Part model, mm, in its own coordinate system. Face numbers are marked on the shaded views. A direction names the side the tool comes from. Give positions to 0.01 mm unless a question says otherwise; leave off trailing zeros. Order: outer loops, then holes, each group sorted by start corner. A loop starts at its lowest first (then second) coordinate and runs counter-clockwise, first axis right, second up.
1. Drop flat-ended pins along their axis: pin 1 Ø2.5 at (x, z) = (-26.5, 0) entering from -Y; pin 2 Ø8 at (x, z) = (1, 2.5) entering from -Y; pin 3 Ø1.5 at (y, z) = (4, -1.5) entering from -X; pin 4 Ø4 at (x, z) = (-13.25, -22.95) entering from +Y. Give the stop position or say it passes through.
2. Slice it at A-A on y = 2. Give the number of separate pieces and of enclosed holes in the cut face, and give its area (3 significant figures).
3. Slice it at B-B on x = -26.5. List the corners of the cut face in (y, z).
4. Mould opens along X. For the marked faces 1 and 2 say: +X half, -X half, draft (parallel to the pull), parting line (faces both ways), or undercut.
5. Slice it at C-C on x = 4.5. List the corners of the cut face in (y, z), and give its area (3 significant figures).
6. Which spindle directions (+Z, -Z, +X, -X, +Y, -Y) get a long thin tool onto all of the face, cutting with end or side? Do the marked faces 3 and 4. Say none if no direction does.
7. Slice it at D-D on z = 11.5. List the corners of the cut face in (x, y).
8. Probe line 1 (X direction, y = 1.6, z = 0); line 2 (X direction, y = 1, z = -22); line 3 (X direction, y = 1.5, z = -23.5). List the from-to ranges inside material, lowest first.
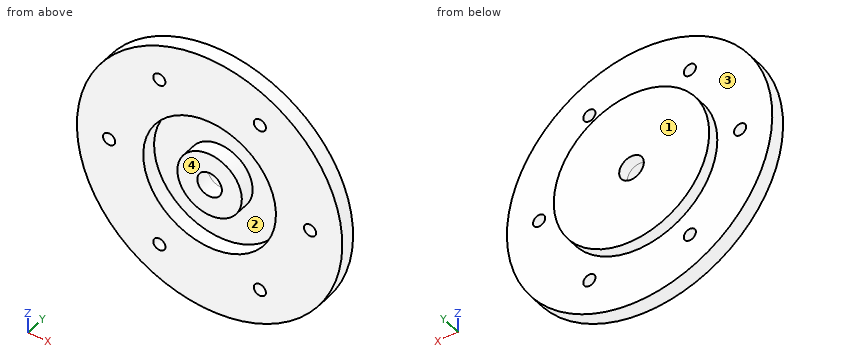
from build123d import *

# Parameters (mm, degrees)
SKETCH_1_R      = 35
SKETCH_1_R_2    = 1.6
SKETCH_1_R_3    = 17.5
EXTRUDE_1_DEPTH = 4
SKETCH_2_R      = 20.5
SKETCH_2_R_2    = 17.5
EXTRUDE_2_DEPTH = 3
EXTRUDE_START   = -3
SKETCH_3_R      = 17.5
SKETCH_3_R_2    = 3.25
EXTRUDE_3_DEPTH = 3
EXTRUDE_START_2 = 4
SKETCH_4_R      = 8.5
SKETCH_4_R_2    = 3.25
EXTRUDE_4_DEPTH = 4


with BuildPart() as part:
    # Эскиз1 → Бобышка-Вытянуть1 (new body)
    with BuildSketch(Plane(origin=(0, 0, 0), x_dir=(1, 0, 0), z_dir=(0, 1, 0))):
        with Locations(Location((0, 0, 0), (0, 0, 270))):
            Circle(SKETCH_1_R)
        with Locations(Location((-13.25, -22.9496732, 0), (0, 0, 270))):
            Circle(SKETCH_1_R_2, mode=Mode.SUBTRACT)
        with Locations(Location((13.25, -22.9496732, 0), (0, 0, 270))):
            Circle(SKETCH_1_R_2, mode=Mode.SUBTRACT)
        with Locations(Location((26.5, 0, 0), (0, 0, 270))):
            Circle(SKETCH_1_R_2, mode=Mode.SUBTRACT)
        with Locations(Location((13.25, 22.9496732, 0), (0, 0, 270))):
            Circle(SKETCH_1_R_2, mode=Mode.SUBTRACT)
        with Locations(Location((-13.25, 22.9496732, 0), (0, 0, 270))):
            Circle(SKETCH_1_R_2, mode=Mode.SUBTRACT)
        with Locations(Location((-26.5, 0, 0), (0, 0, 270))):
            Circle(SKETCH_1_R_2, mode=Mode.SUBTRACT)
        with Locations(Location((0, 0, 0), (0, 0, 270))):
            Circle(SKETCH_1_R_3, mode=Mode.SUBTRACT)
    extrude(amount=EXTRUDE_1_DEPTH)

    # Эскиз2 → Бобышка-Вытянуть2 (add)
    with BuildSketch(Plane(origin=(0, 4, 0), x_dir=(1, 0, 0), z_dir=(0, 1, 0))):
        with Locations(Location((0, 0, 0), (0, 0, 270))):
            Circle(SKETCH_2_R)
        with Locations(Location((0, 0, 0), (0, 0, 270))):
            Circle(SKETCH_2_R_2, mode=Mode.SUBTRACT)
    extrude(amount=EXTRUDE_2_DEPTH)

    # Эскиз3 → Бобышка-Вытянуть3 (add)
    with BuildSketch(Plane(origin=(0, 7, 0), x_dir=(1, 0, 0), z_dir=(0, 1, 0)).offset(EXTRUDE_START)):
        with Locations(Location((0, 0, 0), (0, 0, 270))):
            Circle(SKETCH_3_R)
        with Locations(Location((0, 0, 0), (0, 0, 270))):
            Circle(SKETCH_3_R_2, mode=Mode.SUBTRACT)
    extrude(amount=EXTRUDE_3_DEPTH)

    # Эскиз4 → Бобышка-Вытянуть4 (add)
    with BuildSketch(Plane.XZ.offset(-4).offset(EXTRUDE_START_2)):
        with Locations(Location((0, 0, 0), (0, 0, 90))):
            Circle(SKETCH_4_R)
        with Locations(Location((0, 0, 0), (0, 0, 90))):
            Circle(SKETCH_4_R_2, mode=Mode.SUBTRACT)
    extrude(amount=-EXTRUDE_4_DEPTH)


solid = part.part
Data:
1. pin 1: passes through
1. pin 2: stops at y = 0
1. pin 3: stops at x = -34.99
1. pin 4: stops at y = 4
2. separate pieces: 2
2. enclosed holes: 8
2. area: 3,030 mm2
3. outline: (0, -22.86) - (4, -22.86) - (4, -1.6) - (0, -1.6) - close; (0, 1.6) - (4, 1.6) - (4, 22.86) - (0, 22.86) - close
4. face 1: draft
4. face 2: undercut
5. outline: (0, -34.71) - (4, -34.71) - (4, -20) - (7, -20) - (7, 20) - (4, 20) - (4, 34.71) - (0, 34.71) - (0, 16.91) - (4, 16.91) - (4, 7.21) - (0, 7.21) - (0, -7.21) - (4, -7.21) - (4, -16.91) - (0, -16.91) - close
5. area: 320 mm2
6. face 3: +Y
6. face 4: +Z, -Z, +X, -X, -Y
7. outline: (-33.06, 0) - (-13.19, 0) - (-13.19, 4) - (13.19, 4) - (13.19, 0) - (33.06, 0) - (33.06, 4) - (16.97, 4) - (16.97, 7) - (-16.97, 7) - (-16.97, 4) - (-33.06, 4) - close
8. line 1: x = -35 to -28.1, -24.9 to -17.5, -8.5 to -3.25, 3.25 to 8.5, 17.5 to 24.9, 28.1 to 35
8. line 2: x = -27.22 to -14.54, -11.96 to 11.96, 14.54 to 27.22
8. line 3: x = -25.94 to -14.75, -11.75 to 11.75, 14.75 to 25.94
